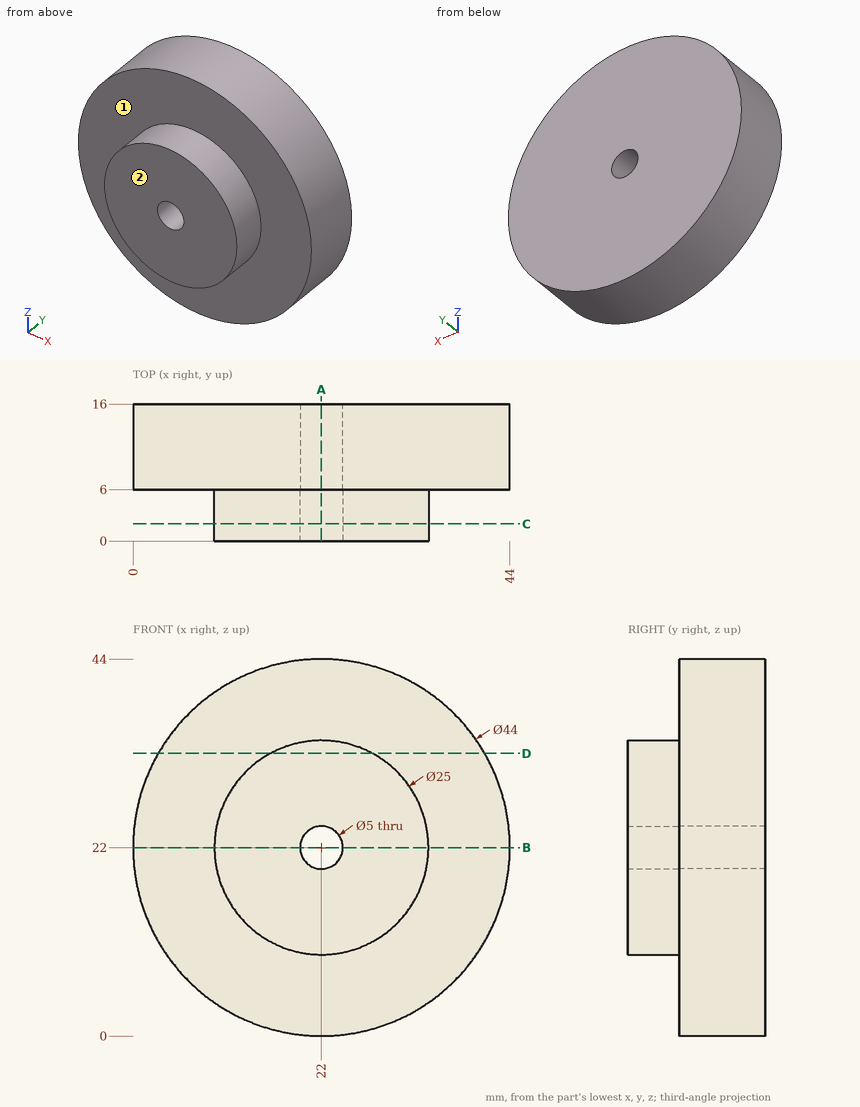
Answer from the drawing. Dimensions are ordinates in mm from the lowest x, y and z of the part. A direction names the side the tool comes from. Give positions to 0.01 mm unless a question says otherwise; leave off trailing zeros. Write each loop counter-clockwise with the first axis right and the second up, starting at its lowest first coordinate (ties: lowest second). Pieces come first, ordered by that corner, then holes.
1) A tool of negligible diameter and unlimited length cuts with its end or side. For the marked faces 1 and 2, from which of +Z, -Z, +X, -X, +Y, -Y can it reach the whole face along a straight path? Write none if from no direction.
2) Section A-A (x = 22) is taken. Write down the section's boundary in (y, z), and give its area (3 significant figures).
3) Find the intervals of material crossed by L1, parallel to Z at x = 22, y = 3.85; L2, parallel to Z at x = 22, y = 11.75; L3, parallel to Y at x = 9, z = 34, in increasing order.
4) Section D-D (z = 33) is taken. Write down the section's boundary in (x, y).
5) Section B-B (z = 22) is taken. Write down the section's boundary in (x, y), and give its area (3 significant figures).
6) Given P1, Ø2, axis at x = 8, y = 5.5, coming from the -Z side; P2, Ø4, axis at y = 2, z = 27, coming from the -X side; P3, Ø8, axis at y = 5, z = 39, coming from the +X side; P4, Ø3, axis at x = 22, z = 22, coming from the +Y side, each flat-ended and moving along its own axis, determine where each tip first touches the part or whether it passes through.
7) Section C-C (y = 2) is taken. Write down the section's boundary in (x, z).
Response:
1. face 1: -Y
1. face 2: +Z, -Z, +X, -X, -Y
2. outline: (0, 9.5) - (6, 9.5) - (6, 0) - (16, 0) - (16, 19.5) - (0, 19.5) - close; (0, 24.5) - (16, 24.5) - (16, 44) - (6, 44) - (6, 34.5) - (0, 34.5) - close
2. area: 510 mm2
3. L1: z = 9.5 to 19.5, 24.5 to 34.5
3. L2: z = 0 to 19.5, 24.5 to 44
3. L3: y = 6 to 16
4. outline: (2.95, 6) - (16.06, 6) - (16.06, 0) - (27.94, 0) - (27.94, 6) - (41.05, 6) - (41.05, 16) - (2.95, 16) - close
5. outline: (0, 6) - (9.5, 6) - (9.5, 0) - (19.5, 0) - (19.5, 16) - (0, 16) - close; (24.5, 0) - (34.5, 0) - (34.5, 6) - (44, 6) - (44, 16) - (24.5, 16) - close
5. area: 510 mm2
6. P1: stops at z = 4.35
6. P2: stops at x = 9.87
6. P3: stops at x = 39.65
6. P4: passes through
7. outline: circle Ø25 at (22, 22); hole circle Ø5 at (22, 22)
